```python
from build123d import *

# Parameters (mm, degrees)
SKETCH2_W           = 49
SKETCH2_H           = 58
BOSS_EXTRUDE1_DEPTH = 3
SKETCH3_W           = 29
SKETCH3_H           = 38
CUT_EXTRUDE1_DEPTH  = 3
SKETCH4_W           = 20
SKETCH4_H           = 3
BOSS_EXTRUDE2_DEPTH = 10
SKETCH5_W           = 3
SKETCH5_H           = 20
BOSS_EXTRUDE3_DEPTH = 16
SKETCH7_W           = 20
SKETCH7_H           = 3
BOSS_EXTRUDE4_DEPTH = 30


with BuildPart() as part:
    # Sketch2 → Boss-Extrude1 (new body)
    with BuildSketch(Plane(origin=(0, 0, 0), x_dir=(1, 0, 0), z_dir=(0, 1, 0))):
        Rectangle(SKETCH2_W, SKETCH2_H)
    extrude(amount=BOSS_EXTRUDE1_DEPTH)

    # Sketch3 → Cut-Extrude1 (cut)
    with BuildSketch(Plane(origin=(0, 3, 0), x_dir=(1, 0, 0), z_dir=(0, 1, 0))):
        Rectangle(SKETCH3_W, SKETCH3_H)
    extrude(amount=-CUT_EXTRUDE1_DEPTH, mode=Mode.SUBTRACT)

    # Sketch4 → Boss-Extrude2 (add)
    with BuildSketch(Plane.ZY.offset(24.5)):
        with Locations((0, 1.5)):
            Rectangle(SKETCH4_W, SKETCH4_H)
    boss_extrude2 = extrude(amount=BOSS_EXTRUDE2_DEPTH)

    # Sketch5 → Boss-Extrude3 (add)
    with BuildSketch(Plane(origin=(0, 3, 0), x_dir=(1, 0, 0), z_dir=(0, 1, 0))):
        with Locations((-33, 0)):
            Rectangle(SKETCH5_W, SKETCH5_H)
    boss_extrude3 = extrude(amount=BOSS_EXTRUDE3_DEPTH)

    # Sketch7 → Boss-Extrude4 (add)
    with BuildSketch(Plane.ZY.offset(34.5)):
        with Locations((0, 17.5)):
            Rectangle(SKETCH7_W, SKETCH7_H)
    boss_extrude4 = extrude(amount=BOSS_EXTRUDE4_DEPTH)

    # Mirror1: Boss-Extrude2, Boss-Extrude3, Boss-Extrude4 across plane
    add(boss_extrude2.mirror(Plane(origin=(0, 0, 0), x_dir=(0, 0, 1), z_dir=(1, 0, 0))))
    add(boss_extrude3.mirror(Plane(origin=(0, 0, 0), x_dir=(0, 0, 1), z_dir=(1, 0, 0))))
    add(boss_extrude4.mirror(Plane(origin=(0, 0, 0), x_dir=(0, 0, 1), z_dir=(1, 0, 0))))


solid = part.part
```
Geometry check sheet. Reference: the model listing, model coordinates, mm. A direction names the side the tool comes from. Coordinates: 2 decimals unless noted, no trailing zeros. Order: outer loops, then holes, each group sorted by start corner. A loop starts at its lowest first (then second) coordinate and runs counter-clockwise, first axis right, second up. Notation, with made-up numbers: (0.5, 23.5) - (21.5, 23.5) arc R6 ccw to (21.5, 31.5) - close; hole circle Ø11 at (9, 66.25). An arc over 180 degrees is marked (long way). Answer as a JSON object with one key per item and string values. Group by question number.
Item 1: Tool access check on faces 4 (the face through (0, 2, 19)), 5 (the face through (-40, 16.5, 10)), 6 (the face through (-40, 16.5, -10)), 7 (the face through (24.5, 1, -19)), 8 (the face through (0, 3, -20)). Record the directions out of +Z, -Z, +X, -X, +Y, -Y that give a thin tool (end or side, any length) a straight path to the whole face; none if there is none.
Item 2: Sectioned sample at C-C, the plane x = 4.5. Record the cut outline in (y, z), and give its area (3 significant figures).
Item 3: Sectioned sample at A-A, the plane y = 13.5. Record the cut outline in (x, z).
Item 4: Draft check along Z on faces 1 (the face through (14.5, 2, 0)), 2 (the face through (48, 19, 0)), 3 (the face through (0, 1, -29)). Enter one of: +Z half, -Z half, draft (parallel to the pull), parting line (faces both ways), or undercut.
Item 5: Scan lines: probe 1 along X at (y, z) = (15.75, -6.5); probe 2 along X at (y, z) = (17.75, -1.5); probe 3 along Y at (x, z) = (-27, 2). Record each from-to range of solid material in increasing order.
Item 6: Sectioned sample at B-B, the plane z = 5. Record the cut outline in (x, y), and give its area (3 significant figures).
Item 7: Sectioned sample at D-D, the plane x = 29. Record the cut outline in (y, z), and give its area (3 significant figures).
Item 8: Depth check by flat-ended pin: pin 1 Ø0.9 at (y, z) = (1, -21) entering from -X; pin 2 Ø5 at (y, z) = (6, 15) entering from +X; pin 3 Ø3.5 at (y, z) = (2, -15) entering from +X; pin 4 Ø16 at (x, z) = (45, -4.5) entering from -Y. Enter the tip coordinate at first touch or a pass-through.
Resolved:
{
 "1": {"face 4": "+Y, -Y", "face 5": "+Z, -X, +Y, -Y", "face 6": "-Z, -X, +Y, -Y", "face 7": "-Z, +X, +Y, -Y", "face 8": "+Z, -Z, +Y"},
 "2": {"outline": "(0, -29) - (3, -29) - (3, -19) - (0, -19) - close; (0, 19) - (3, 19) - (3, 29) - (0, 29) - close", "area": "60.0 mm^2"},
 "3": {"outline": "(-34.5, -10) - (-31.5, -10) - (-31.5, 10) - (-34.5, 10) - close; (31.5, -10) - (34.5, -10) - (34.5, 10) - (31.5, 10) - close"},
 "4": {"face 1": "undercut", "face 2": "draft", "face 3": "-Z half"},
 "5": {"probe 1": "-34.5 to -31.5, 31.5 to 34.5", "probe 2": "-64.5 to -31.5, 31.5 to 64.5", "probe 3": "0 to 3"},
 "6": {"outline": "(-64.5, 16) - (-34.5, 16) - (-34.5, 0) - (-14.5, 0) - (-14.5, 3) - (-31.5, 3) - (-31.5, 19) - (-64.5, 19) - close; (14.5, 0) - (34.5, 0) - (34.5, 16) - (64.5, 16) - (64.5, 19) - (31.5, 19) - (31.5, 3) - (14.5, 3) - close", "area": "396 mm^2"},
 "7": {"outline": "(0, -10) - (3, -10) - (3, 10) - (0, 10) - close", "area": "60.0 mm^2"},
 "8": {"pin 1": "x = -24.5", "pin 2": "through", "pin 3": "x = 24.5", "pin 4": "y = 16"}
}
